The figure shows three views and two pictorial views of one solid part (mm, origin at its lowest corner). Answer the questions. A direction names the side the tool comes from. Round coordinates to 2 decimals unless told otherwise and drop trailing zeros. Use a Markdown table: item, result. Add a question column.
Q1. Consider line 1 (Z direction, x = 28, y = 7); line 2 (X direction, y = 2.25, z = 24.5); line 3 (Z direction, x = 31, y = 5) (1 decimal). Determine where each line is inside the solid, lowest interval first.
Q2. Given pin 1 Ø6 at (y, z) = (10, 35.5) entering from -X; pin 2 Ø1.5 at (y, z) = (6, 31.5) entering from +X (1 decimal); pin 3 Ø1.5 at (y, z) = (3.5, 29.5) entering from +X; pin 4 Ø8 at (x, z) = (47.5, 11) entering from +Y, each flat-ended and moving along its own axis, determine where each tip first touches the part or whether it passes through.
Q3. For a pull along Z with two mould halves and no side action, classify the marked faces 1, 2 and 3 as released by +Z, released by -Z, zero draft, split by the parting line, or undercut.
Q4. Section A-A on y = 11.25 is taken. Give the number of separate pieces and of enclosed holes in the cut face.
Q5. Which of the six approach directions +Z, -Z, +X, -X, +Y, -Y give full straight-line access (tool end or side, diameter ignored) to the marked faces 4 and 5?
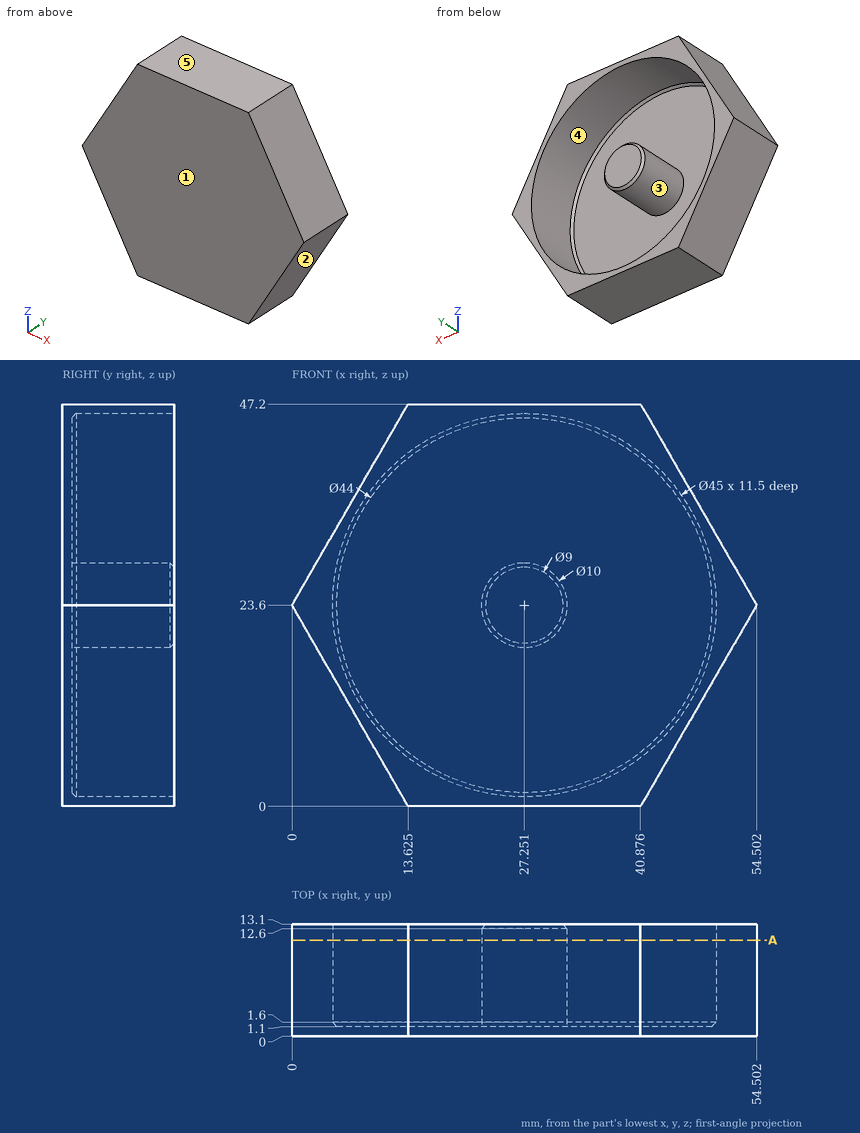
Checked values:
| question | item | result |
|---|---|---|
| 1 | line 1 | z = 0 to 1.11, 18.66 to 28.54, 46.09 to 47.2 |
| 1 | line 2 | x = 0.52 to 4.77, 22.33 to 32.17, 49.73 to 53.98 |
| 1 | line 3 | z = 0 to 1.4, 20.3 to 26.9, 45.8 to 47.2 |
| 2 | pin 1 | stops at x = 5.14 |
| 2 | pin 2 | stops at x = 50.4 |
| 2 | pin 3 | stops at x = 51.53 |
| 2 | pin 4 | stops at y = 13.1 |
| 3 | face 1 | zero draft |
| 3 | face 2 | released by -Z |
| 3 | face 3 | undercut |
| 4 | separate pieces | 2 |
| 4 | enclosed holes | 1 |
| 5 | face 4 | +Y |
| 5 | face 5 | +Z, +X, -X, +Y, -Y |
